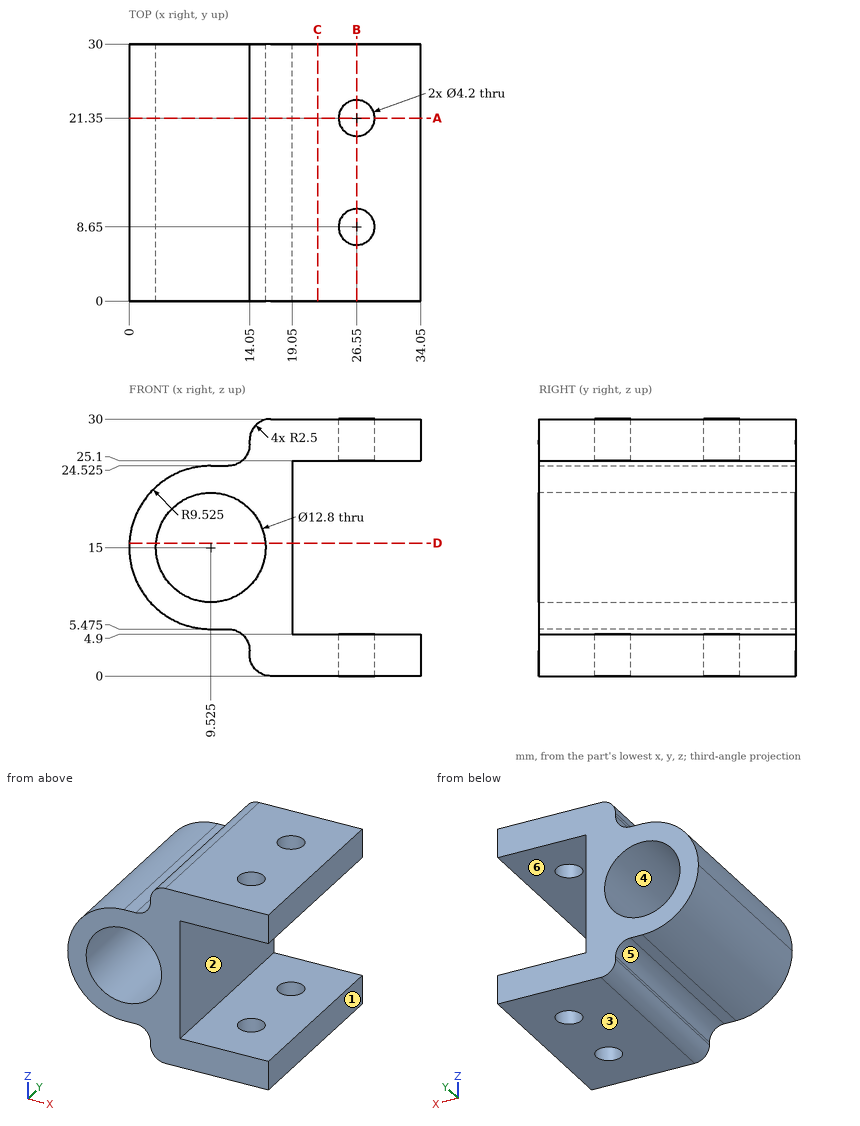
Check sheet for the drawn part. Datum: minimum x, y, z corner. Units: mm. A direction names the side the tool comes from. Coordinates: 2 decimals unless noted, no trailing zeros. Loops run counter-clockwise (first coordinate to the right, second up) from the corner with the lowest first, then second, coordinate; pieces in that order, holes last. Notation, with made-up numbers: M -7.5,-6 L 7.5,-6 A32 ccw 7.5,31 Z; hole C -10.75,-33.5 d6. An arc over 180 degrees is marked long. Answer as a JSON object with one key per item and string values.
1. Access from +Z, -Z, +X, -X, +Y, -Y to the whole of each face (thin tool, end or side, straight path). Record for the marked faces 5 and 6.
Outcome:
{"face 5": "-Z, -X, +Y, -Y", "face 6": "+X, +Y, -Y"}
2. Sectioned sample at D-D on z = 15.5. Record the cut outline in (x, y).
Outcome:
{"outline": "M 0.01,0 L 3.14,0 L 3.14,30 L 0.01,30 Z; M 15.91,0 L 19.05,0 L 19.05,30 L 15.91,30 Z"}
3. Depth check by flat-ended pin: P1, Ø4, axis at y = 25, z = 12, coming from the -X side; P2, Ø5, axis at y = 17.5, z = 11, coming from the +X side; P3, Ø0.6, axis at x = 10, y = 21, coming from the -Z side (3 decimals). Enter the tip coordinate at first touch or a pass-through.
Outcome:
{"P1": "x = 0.05", "P2": "x = 19.05", "P3": "z = 5.475"}
4. Sectioned sample at C-C on x = 22. Record the cut outline in (y, z), and give its area (3 significant figures).
Outcome:
{"outline": "M 0,0 L 30,0 L 30,4.9 L 0,4.9 Z; M 0,25.1 L 30,25.1 L 30,30 L 0,30 Z", "area": "294 mm²"}
5. Release check for a two-part mould opening along Z. For the marked faces 1, 2, 3 and 4 record: pulls with the +Z half, pulls with the -Z half, needs draft (parallel to the pull), parting line crosses it, or undercut.
Outcome:
{"face 1": "needs draft", "face 2": "undercut", "face 3": "pulls with the -Z half", "face 4": "undercut"}
6. Scan lines: L1, parallel to Z at x = 29.5, y = 23.25; L2, parallel to Y at x = 26, z = 3; L3, parallel to X at y = 9, z = 19. Record each from-to range of solid material in increasing order. Write a range as from..to.
Outcome:
{"L1": "0..4.9, 25.1..30", "L2": "0..6.62, 10.68..19.32, 23.38..30", "L3": "0.88..4.53, 14.52..19.05"}
7. Sectioned sample at B-B on x = 26.55. Record the cut outline in (y, z).
Outcome:
{"outline": "M 0,0 L 6.55,0 L 6.55,4.9 L 0,4.9 Z; M 0,25.1 L 6.55,25.1 L 6.55,30 L 0,30 Z; M 10.75,0 L 19.25,0 L 19.25,4.9 L 10.75,4.9 Z; M 10.75,25.1 L 19.25,25.1 L 19.25,30 L 10.75,30 Z; M 23.45,0 L 30,0 L 30,4.9 L 23.45,4.9 Z; M 23.45,25.1 L 30,25.1 L 30,30 L 23.45,30 Z"}
8. Sectioned sample at A-A on y = 21.35. Record the cut outline in (x, z) (3 decimals).
Outcome:
{"outline": "M 9.525,5.475 L 11.55,5.475 A2.5 cw 14.05,2.975 L 14.05,2.5 A2.5 ccw 16.55,0 L 24.45,0 L 24.45,4.9 L 19.05,4.9 L 19.05,25.1 L 24.45,25.1 L 24.45,30 L 16.55,30 A2.5 ccw 14.05,27.5 L 14.05,27.025 A2.5 cw 11.55,24.525 L 9.525,24.525 A9.525 ccw Z; M 28.65,0 L 34.05,0 L 34.05,4.9 L 28.65,4.9 Z; M 28.65,25.1 L 34.05,25.1 L 34.05,30 L 28.65,30 Z; hole C 9.525,15 d12.8"}
